For this review, take the finished solid that the model builds, in its own axes (mm). Face numbers are marked on the shaded views. Coordinates: 2 decimals unless noted, no trailing zeros. Loops run counter-clockwise (first coordinate to the right, second up) from the corner with the lowest first, then second, coordinate; pieces in that order, holes last. Notation, with made-up numbers: (-9, 75.25) -> (6, 75.25) arc R29 cw to (6, 104.25) -> close; hole circle Ø9 at (-23, 74.5). An arc over 180 degrees is marked (long way). One line per item, written item: value.
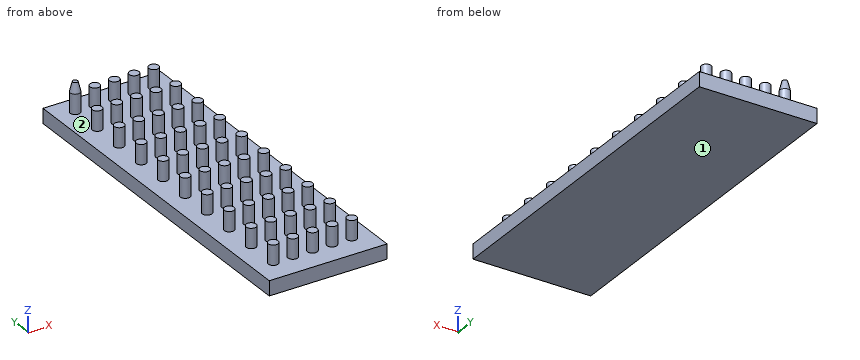
from build123d import *

# Parameters (mm, degrees)
F0_W     = 152.4
F0_H     = 19.05
F1_DEPTH = 457.2
F2_R     = 6.35
F3_DEPTH = 25.4
F4_R     = 6.35
F6_R     = 3.175


with BuildPart() as f1:
    # F0 (on Front) → F1 (new body)
    with BuildSketch(Plane.XZ):
        with Locations((76.2, -9.525)):
            Rectangle(F0_W, F0_H)
    extrude(amount=F1_DEPTH)

    # F2 (on face) → F3 (join)
    with BuildSketch(Plane.XY):
        with Locations((25.4, -25.4)):
            Circle(F2_R)
        with Locations((25.4, -69.85)):
            Circle(F2_R)
        with Locations((25.4, -114.3)):
            Circle(F2_R)
        with Locations((25.4, -158.75)):
            Circle(F2_R)
        with Locations((25.4, -203.2)):
            Circle(F2_R)
        with Locations((25.4, -247.65)):
            Circle(F2_R)
        with Locations((25.4, -292.1)):
            Circle(F2_R)
        with Locations((25.4, -336.55)):
            Circle(F2_R)
        with Locations((50.8, -25.4)):
            Circle(F2_R)
        with Locations((50.8, -69.85)):
            Circle(F2_R)
        with Locations((50.8, -114.3)):
            Circle(F2_R)
        with Locations((50.8, -158.75)):
            Circle(F2_R)
        with Locations((50.8, -203.2)):
            Circle(F2_R)
        with Locations((50.8, -247.65)):
            Circle(F2_R)
        with Locations((50.8, -292.1)):
            Circle(F2_R)
        with Locations((50.8, -336.55)):
            Circle(F2_R)
        with Locations((76.2, -25.4)):
            Circle(F2_R)
        with Locations((76.2, -69.85)):
            Circle(F2_R)
        with Locations((76.2, -114.3)):
            Circle(F2_R)
        with Locations((76.2, -158.75)):
            Circle(F2_R)
        with Locations((76.2, -203.2)):
            Circle(F2_R)
        with Locations((76.2, -247.65)):
            Circle(F2_R)
        with Locations((76.2, -292.1)):
            Circle(F2_R)
        with Locations((76.2, -336.55)):
            Circle(F2_R)
        with Locations((101.6, -25.4)):
            Circle(F2_R)
        with Locations((101.6, -69.85)):
            Circle(F2_R)
        with Locations((101.6, -114.3)):
            Circle(F2_R)
        with Locations((101.6, -158.75)):
            Circle(F2_R)
        with Locations((101.6, -203.2)):
            Circle(F2_R)
        with Locations((101.6, -247.65)):
            Circle(F2_R)
        with Locations((101.6, -292.1)):
            Circle(F2_R)
        with Locations((101.6, -336.55)):
            Circle(F2_R)
        with Locations((127, -25.4)):
            Circle(F2_R)
        with Locations((127, -69.85)):
            Circle(F2_R)
        with Locations((127, -114.3)):
            Circle(F2_R)
        with Locations((127, -158.75)):
            Circle(F2_R)
        with Locations((127, -203.2)):
            Circle(F2_R)
        with Locations((127, -247.65)):
            Circle(F2_R)
        with Locations((127, -292.1)):
            Circle(F2_R)
        with Locations((127, -336.55)):
            Circle(F2_R)
        with Locations((25.4, -381)):
            Circle(F2_R)
        with Locations((25.4, -425.45)):
            Circle(F2_R)
        with Locations((50.8, -381)):
            Circle(F2_R)
        with Locations((50.8, -425.45)):
            Circle(F2_R)
        with Locations((76.2, -381)):
            Circle(F2_R)
        with Locations((76.2, -425.45)):
            Circle(F2_R)
        with Locations((101.6, -381)):
            Circle(F2_R)
        with Locations((101.6, -425.45)):
            Circle(F2_R)
        with Locations((127, -381)):
            Circle(F2_R)
        with Locations((127, -425.45)):
            Circle(F2_R)
    extrude(amount=F3_DEPTH)

    # F4 (on face) → F7 section 0
    with BuildSketch(Plane.XY.offset(25.4)):
        with Locations((25.4, -25.4)):
            Circle(F4_R)
    # F6 (on offset) → F7 section 1
    with BuildSketch(Plane.XY.offset(38.1)):
        with Locations((25.4, -25.4)):
            Circle(F6_R)
    loft()


solid = f1.part
1. The part is to be moulded in two halves that separate along Y. For the marked faces 1 and 2, say which applies: pulls with the +Y half, pulls with the -Y half, needs draft (parallel to the pull), parting line crosses it, or undercut.
Return value:
face 1: needs draft
face 2: undercut
2. Take a section at D-D, the plane z = 34. Give the boundary of the cut face in (x, y).
Return value:
outline: circle Ø8.4 at (25.4, -25.4)
3. Take a section at C-C, the plane x = 39. Give the boundary of the cut face in (y, z), and give its area (3 significant figures).
Return value:
outline: (-457.2, -19.05) -> (0, -19.05) -> (0, 0) -> (-457.2, 0) -> close
area: 8,710 mm2
4. Insertion check: pin 1 Ø4 at (x, y) = (125, -72.5) entering from +Z; pin 2 Ø5 at (x, y) = (24.5, -132.5) entering from +Z; pin 3 Ø1 at (x, z) = (50, 3.5) entering from +Y; pin 4 Ø4 at (y, z) = (-119.5, -8.5) entering from -X. Each pin has a flat end and moves straight along its axis. Give the tip position at first contact, or say it passes through.
Return value:
pin 1: stops at z = 25.4
pin 2: stops at z = 0
pin 3: stops at y = -19.06
pin 4: stops at x = 0
5. To check wall thickness, follow probe 1 along Z at (x, y) = (98, -141); probe 2 along X at (y, z) = (-31, 4); probe 3 along Z at (x, y) = (103.5, -69.5). State the ranges of each line that lie inside material, in increasing order. Write a range as from..to.
Return value:
probe 1: z = -19.05..0
probe 2: x = 22.41..28.39, 47.81..53.79, 73.21..79.19, 98.61..104.59, 124.01..129.99
probe 3: z = -19.05..25.4
6. Take a section at B-B, the plane z = 6. Give the number of separate pieces and of enclosed holes in the cut face, and give its area (3 significant figures).
Return value:
separate pieces: 50
enclosed holes: 0
area: 6,330 mm2
7. Take a section at A-A, the plane y = -69.85. Give the boundary of the cut face in (x, z), and give its area (3 significant figures).
Return value:
outline: (0, -19.05) -> (152.4, -19.05) -> (152.4, 0) -> (133.35, 0) -> (133.35, 25.4) -> (120.65, 25.4) -> (120.65, 0) -> (107.95, 0) -> (107.95, 25.4) -> (95.25, 25.4) -> (95.25, 0) -> (82.55, 0) -> (82.55, 25.4) -> (69.85, 25.4) -> (69.85, 0) -> (57.15, 0) -> (57.15, 25.4) -> (44.45, 25.4) -> (44.45, 0) -> (31.75, 0) -> (31.75, 25.4) -> (19.05, 25.4) -> (19.05, 0) -> (0, 0) -> close
area: 4,520 mm2
